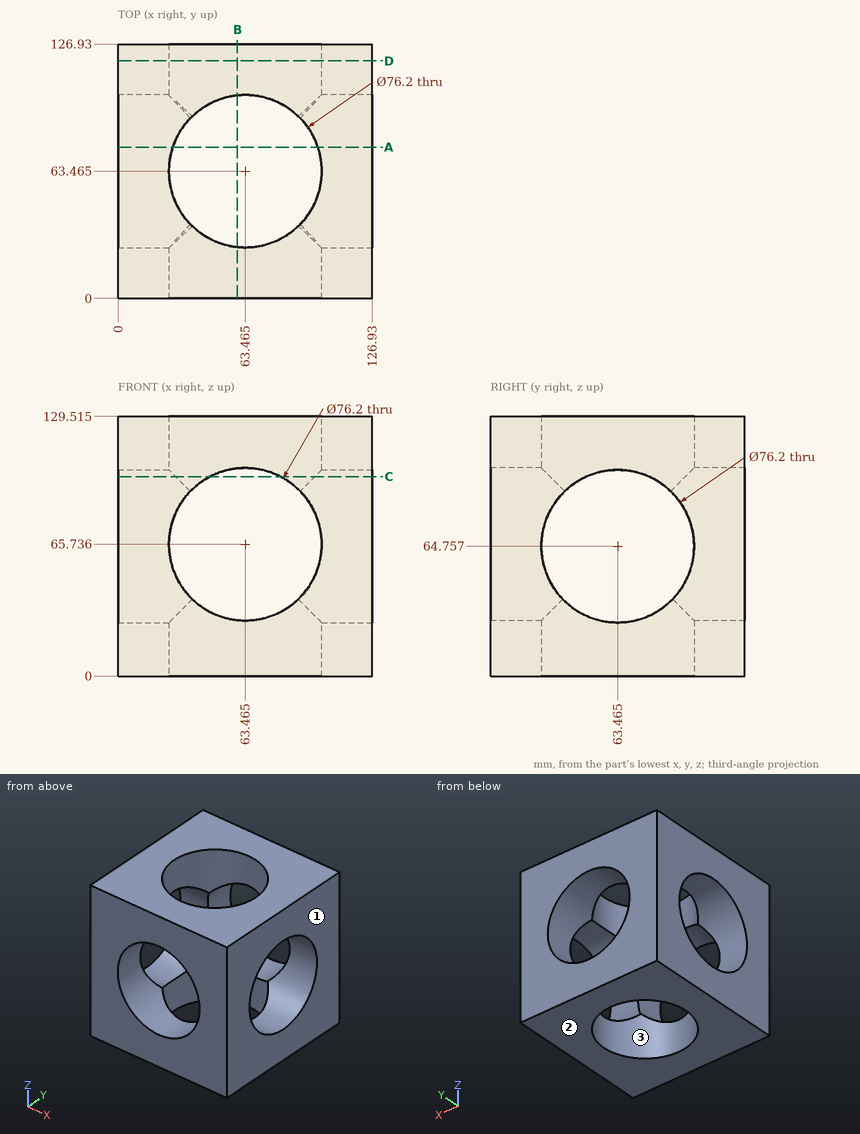
The figure shows three views and two pictorial views of one solid part (mm, origin at its lowest corner). Answer the questions. Give positions to 0.01 mm unless a question says otherwise; leave off trailing zeros. Write each loop counter-clockwise with the first axis right and the second up, starting at its lowest first coordinate (ties: lowest second). Pieces come first, ordered by that corner, then holes. Notation, with made-up numbers: M 78.5,29.25 L 137.5,29.25 A23 cw 137.5,54.25 Z; hole C 73.25,29.25 d4. An arc over 180 degrees is marked long. One line per item, written item: value. Start each with the question number.
(1) Find section C-C (z = 99.5). Determine the outline of the cut face in (x, y) (1 decimal).
(2) Find the intervals of material crossed by line 1 (Z direction, x = 117, y = 65) (1 decimal); line 2 (Y direction, x = 9, z = 75.5); line 3 (X direction, y = 101, z = 90.5), in increasing order.
(3) Find section D-D (y = 118.5). Determine the outline of the cut face in (x, z) (1 decimal).
(4) Find section A-A (y = 75.5). Determine the outline of the cut face in (x, z) (1 decimal).
(5) Find section B-B (x = 59.5). Determine the outline of the cut face in (y, z) (1 decimal), plus the area to 3 significant figures.
(6) Determine the mould class of the marked faces 1, 2 and 3 for opening direction X: pulls with the +X half, pulls with the -X half, needs draft (parallel to the pull), parting line crosses it, or undercut.
Results below:
1. outline: M 0,0 L 45.8,0 L 45.8,29.7 A38.1 cw 28.7,47.8 L 0,47.8 Z; M 0,79.1 L 28.7,79.1 A38.1 cw 45.8,97.2 L 45.8,126.9 L 0,126.9 Z; M 81.1,0 L 126.9,0 L 126.9,47.8 L 98.2,47.8 A38.1 cw 81.1,29.7 Z; M 81.1,97.2 A38.1 cw 98.2,79.1 L 126.9,79.1 L 126.9,126.9 L 81.1,126.9 Z
2. line 1: z = 0 to 26.7, 102.8 to 129.5
2. line 2: y = 0 to 26.91, 100.02 to 126.93
2. line 3: x = 0 to 34.51, 92.42 to 126.93
3. outline: M 0,0 L 126.9,0 L 126.9,129.5 L 0,129.5 Z; hole C 63.5,65.7 d76.2
4. outline: M 0,0 L 27.3,0 L 27.3,28.6 L 0,28.6 Z; M 0,100.9 L 27.3,100.9 L 27.3,129.5 L 0,129.5 Z; M 99.6,0 L 126.9,0 L 126.9,28.6 L 99.6,28.6 Z; M 99.6,100.9 L 126.9,100.9 L 126.9,129.5 L 99.6,129.5 Z
5. outline: M 0,0 L 25.6,0 L 25.6,27.8 L 0,27.8 Z; M 0,103.6 L 25.6,103.6 L 25.6,129.5 L 0,129.5 Z; M 101.4,0 L 126.9,0 L 126.9,27.8 L 101.4,27.8 Z; M 101.4,103.6 L 126.9,103.6 L 126.9,129.5 L 101.4,129.5 Z
5. area: 2,750 mm^2
6. face 1: pulls with the +X half
6. face 2: needs draft
6. face 3: undercut
